from build123d import *

# Parameters (mm, degrees)
SKETCH1_W           = 44
SKETCH1_H           = 137
SKETCH1_R           = 2.5
SKETCH1_R_2         = 2
BOSS_EXTRUDE1_DEPTH = 10
SKETCH2_W           = 62
SKETCH2_H           = 4
CUT_EXTRUDE1_DEPTH  = 83.025910541


with BuildPart() as part:
    # Sketch1 → Boss-Extrude1 (new body)
    with BuildSketch(Plane(origin=(0, 0, 0), x_dir=(1, 0, 0), z_dir=(0, 1, 0))):
        Rectangle(SKETCH1_W, SKETCH1_H)
        with Locations(Location((-14, 59.5, 0), (0, 0, 270))):
            Circle(SKETCH1_R, mode=Mode.SUBTRACT)
        with Locations(Location((14, 59.5, 0), (0, 0, 270))):
            Circle(SKETCH1_R, mode=Mode.SUBTRACT)
        with Locations(Location((14, 15.5, 0), (0, 0, 270))):
            Circle(SKETCH1_R, mode=Mode.SUBTRACT)
        with Locations(Location((-14, 15.5, 0), (0, 0, 270))):
            Circle(SKETCH1_R, mode=Mode.SUBTRACT)
        with Locations(Location((14, -13.5, 0), (0, 0, 270))):
            Circle(SKETCH1_R, mode=Mode.SUBTRACT)
        with Locations(Location((-14, -13.5, 0), (0, 0, 270))):
            Circle(SKETCH1_R, mode=Mode.SUBTRACT)
        with Locations(Location((-14, -49.5, 0), (0, 0, 270))):
            Circle(SKETCH1_R, mode=Mode.SUBTRACT)
        with Locations(Location((14, -49.5, 0), (0, 0, 270))):
            Circle(SKETCH1_R, mode=Mode.SUBTRACT)
        with Locations(Location((-16, 1.5, 0), (0, 0, 270))):
            Circle(SKETCH1_R_2, mode=Mode.SUBTRACT)
        with Locations(Location((16, 1.5, 0), (0, 0, 270))):
            Circle(SKETCH1_R_2, mode=Mode.SUBTRACT)
        with Locations(Location((-16, -64.5, 0), (0, 0, 270))):
            Circle(SKETCH1_R_2, mode=Mode.SUBTRACT)
        with Locations(Location((16, -64.5, 0), (0, 0, 270))):
            Circle(SKETCH1_R_2, mode=Mode.SUBTRACT)
    extrude(amount=BOSS_EXTRUDE1_DEPTH)

    # Sketch2 → Cut-Extrude1 (cut, through all)
    with BuildSketch(Plane(origin=(22, 0, 0), x_dir=(0, 0, -1), z_dir=(1, 0, 0))):
        with Locations((37.5, 8)):
            Rectangle(SKETCH2_W, SKETCH2_H)
    extrude(amount=-CUT_EXTRUDE1_DEPTH, mode=Mode.SUBTRACT)


solid = part.part
Design review of the part built by this model. Coordinates are the model's own, in mm. A direction names the side the tool comes from. Round coordinates to 2 decimals unless told otherwise and drop trailing zeros. Order: outer loops, then holes, each group sorted by start corner. A loop starts at its lowest first (then second) coordinate and runs counter-clockwise, first axis right, second up. Notation, with made-up numbers: M -27.5,-39 L 17.5,-39 A32 ccw 17.5,-12 Z; hole C 20.5,83 d10. An arc over 180 degrees is marked long. Answer as CSV lines item,"result". Start each with the question number.
1) Wall thickness on line 1 along X through (y, z) = (3.05, -15.5); line 2 along X through (y, z) = (2.25, -1.5); line 3 along Z through (x, y) = (17, 8.5): over which ranges is each line inside the solid? List them lowest first. Write a range as [from, to].
2) For pin 1 Ø3 at (x, y) = (-10.5, 8.5) entering from -Z; pin 2 Ø6 at (x, z) = (14, -59.5) entering from +Y, all flat-tipped, find the tip position at first contact; note any pin that passes through.
3) Add section C-C (x = 1). Give the boundary of the cut face in (y, z), then the cut area to 3 significant figures.
4) Add section B-B (z = -1.5). Give the boundary of the cut face in (x, y).
5) Tool access review of faces 1 (the face through (13.04, 2.96, -57.19)), 2 (the face through (0, 6, -37)): name each direction out of +Z, -Z, +X, -X, +Y, -Y from which nothing blocks a thin tool from reaching the whole face with its end or side.
6) Add section A-A (z = -59.5). Give the boundary of the cut face in (x, y).
7) The part is to be moulded in two halves that separate along Z. For faces 3 (the face through (-14.017, 4.93, -1.76)), 4 (the face through (-22, 4, 16)), 5 (the face through (0, 8, -6.5)), say which applies: +Z half, -Z half, draft (parallel to the pull), parting line (faces both ways), or undercut.
Resolved:
1,line 1,"[-22, -16.5], [-11.5, 11.5], [16.5, 22]"
1,line 2,"[-22, -18], [-14, 14], [18, 22]"
1,line 3,"[-6.5, -3.23], [0.23, 62.77], [66.23, 68.5]"
2,pin 1,"z = -6.5"
2,pin 2,"y = 6"
3,outline,"M 0,-68.5 L 6,-68.5 L 6,-6.5 L 10,-6.5 L 10,68.5 L 0,68.5 Z"
3,area,"1,120 mm^2"
4,outline,"M -22,0 L -18,0 L -18,10 L -22,10 Z; M -14,0 L 14,0 L 14,10 L -14,10 Z; M 18,0 L 22,0 L 22,10 L 18,10 Z"
5,face 1,"+Y, -Y"
5,face 2,"-Z, +X, -X, +Y"
6,outline,"M -22,0 L -16.5,0 L -16.5,6 L -22,6 Z; M -11.5,0 L 11.5,0 L 11.5,6 L -11.5,6 Z; M 16.5,0 L 22,0 L 22,6 L 16.5,6 Z"
7,face 3,"undercut"
7,face 4,"draft"
7,face 5,"-Z half"
